The model under review builds one solid part; all positions refer to its coordinate system, in mm. A direction names the side the tool comes from. Round coordinates to 2 decimals unless told otherwise and drop trailing zeros. Order: outer loops, then holes, each group sorted by start corner. A loop starts at its lowest first (then second) coordinate and runs counter-clockwise, first axis right, second up. Notation, with made-up numbers: M -11.75,69.25 L 31.25,69.25 A25 cw 31.25,93.25 Z; hole C -18.75,-19 d9. An arc over 180 degrees is marked long. One line per item, written item: value. Start each with the question number.
from build123d import *

# Parameters (mm, degrees)
BOSS_EXTRUDE1_DEPTH     = 9
CUT_EXTRUDE1_DEPTH      = 18.867568385
CUT_EXTRUDE1_DEPTH_BACK = 18.867568385
CHAMFER1_SIZE           = 1
SKETCH4_R               = 1.25
CUT_EXTRUDE2_DEPTH      = 18.867568385
CUT_EXTRUDE3_START      = 3
SKETCH5_R               = 2.325
CUT_EXTRUDE3_DEPTH      = 10
FILLET2_R               = 2
CHAMFER3_SIZE           = 0.75


with BuildPart() as part:
    # Sketch1 → Boss-Extrude1 (new body)
    with BuildSketch(Plane.XY):
        with BuildLine():
            Line((-14, 0.5), (-14, 6.5))
            Line((-14, 6.5), (14, 6.5))
            Line((14, 6.5), (14, 0.5))
            Line((14, 0.5), (3.3, 0))
            ThreePointArc((3.3, 0), (0, 3.3), (-3.3, 0))
            Line((-3.3, 0), (-14, 0.5))
        make_face()
    extrude(amount=BOSS_EXTRUDE1_DEPTH)

    # Sketch2 → Cut-Extrude1 (cut, two sides: drawn at the far end of the back side and taken through both)
    with BuildSketch(Plane.XY.offset(9).offset(-CUT_EXTRUDE1_DEPTH_BACK)):
        Polygon((-10, 5), (0, 6.5), (-14, 6.5), (-14, 1), align=None)
        Polygon((14, 6.5), (0, 6.5), (10, 5), (14, 1), align=None)
    extrude(amount=CUT_EXTRUDE1_DEPTH + CUT_EXTRUDE1_DEPTH_BACK, mode=Mode.SUBTRACT)

    # Chamfer1
    chamfer1_edges = [part.edges().sort_by_distance(p)[0] for p in [
        (14, 0.75, 9),
        (-14, 0.75, 0),
        (-14, 0.75, 9),
        (14, 0.75, 0),
    ]]
    chamfer(chamfer1_edges, length=CHAMFER1_SIZE)

    # Sketch4 → Cut-Extrude2 (cut, through all)
    with BuildSketch(Plane(origin=(0, 0, 0), x_dir=(-1, 0, 0), z_dir=(0, 1, 0))):
        with Locations(Location((-9, 4.5, 0), (0, 0, 216.869897646))):
            Circle(SKETCH4_R)
        with Locations(Location((9, 4.5, 0), (0, 0, 323.130102354))):
            Circle(SKETCH4_R)
    extrude(amount=CUT_EXTRUDE2_DEPTH, mode=Mode.SUBTRACT)

    # Sketch5 → Cut-Extrude3 (cut)
    with BuildSketch(Plane(origin=(0, 0, 0), x_dir=(1, 0, 0), z_dir=(0, 1, 0)).offset(CUT_EXTRUDE3_START)):
        with Locations(Location((9, -4.5, 0), (0, 0, 64.525615739))):
            Circle(SKETCH5_R)
        with Locations(Location((-9, -4.5, 0), (0, 0, 115.474384261))):
            Circle(SKETCH5_R)
    extrude(amount=CUT_EXTRUDE3_DEPTH, mode=Mode.SUBTRACT)

    # Fillet2
    # the kernel refuses this fillet: 2 mm, written as the material it takes off along each edge
    with BuildSketch(Plane(origin=(10, 5, -1.647264498), x_dir=(0.7071067811865476, -0.7071067811865476, 0), z_dir=(0, 0, 1)), Plane(origin=(-10, 5, 4.048306423), x_dir=(-0.7071067811865476, -0.7071067811865476, 0), z_dir=(0, 0, -1))) as fillet2_piece_1:
        with BuildLine():
            CenterArc((FILLET2_R * 0.329452899538, -FILLET2_R), FILLET2_R, 90, 36.46923439)
            Line((-FILLET2_R * 0.264938161546, -FILLET2_R * 0.195823858534), (-FILLET2_R * 0.276825982767, -FILLET2_R * 0.179740335704))
            Line((-FILLET2_R * 0.276825982767, -FILLET2_R * 0.179740335704), (-FILLET2_R * 0.00658905799077, FILLET2_R * 0.02))
            Line((-FILLET2_R * 0.00658905799077, FILLET2_R * 0.02), (FILLET2_R * 0.329452899538, FILLET2_R * 0.02))
            Line((FILLET2_R * 0.329452899538, FILLET2_R * 0.02), (FILLET2_R * 0.329452899538, 0))
        make_face()
    extrude(amount=5.695570921, mode=Mode.SUBTRACT)
    with BuildSketch(Plane(origin=(0, 6.5, 9.75), x_dir=(0.9889363528682978, -0.1483404529302431, 0), z_dir=(0, 0, -1))) as fillet2_piece_2:
        with BuildLine():
            CenterArc((FILLET2_R * 0.15, FILLET2_R), FILLET2_R, 252.93846878, 17.06153122)
            Line((-FILLET2_R * 0.143398533007, FILLET2_R * 0.0440097799511), (-FILLET2_R * 0.149266503667, FILLET2_R * 0.0248899755501))
            Line((-FILLET2_R * 0.149266503667, FILLET2_R * 0.0248899755501), (-FILLET2_R * 0.003, -FILLET2_R * 0.02))
            Line((-FILLET2_R * 0.003, -FILLET2_R * 0.02), (FILLET2_R * 0.15, -FILLET2_R * 0.02))
            Line((FILLET2_R * 0.15, -FILLET2_R * 0.02), (FILLET2_R * 0.15, 0))
        make_face()
    extrude(amount=10.5, mode=Mode.SUBTRACT)
    with BuildSketch(Plane(origin=(-14, 1, -0.95470504), x_dir=(0, -1, 0), z_dir=(0, 0, 1))) as fillet2_piece_3:
        with BuildLine():
            CenterArc((0.861339487, 1.967087638), FILLET2_R, 225, 34.591227114)
            Line((-0.552874076, 0.552874076), (-0.581158347, 0.524589804))
            Line((-0.581158347, 0.524589804), (-0.028284271, -0.028284271))
            Line((-0.028284271, -0.028284271), (0, -0.04))
            ThreePointArc((0, -0.04), (0.25, -0.04), (0.49277321, -0.039341753))
            Line((0.49277321, -0.039341753), (0.5, 0))
        make_face()
    extrude(amount=10.90941008, mode=Mode.SUBTRACT)

    # Chamfer3
    # the kernel refuses this chamfer: 0.75 mm, written as the material it takes off along each edge
    with BuildSketch(Plane(origin=(-14.36384086, 0.63615914, 9), x_dir=(0.7068394360706732, -0.7068394360706737, 0.027495876610586747), z_dir=(0.7071067811865477, 0.7071067811865474, 0))) as chamfer3_piece_1:
        Polygon((CHAMFER3_SIZE * 0.999621916911, CHAMFER3_SIZE * 0.0274958766106), (-CHAMFER3_SIZE * 0.0274958766106, CHAMFER3_SIZE * 0.999621916911), (0, 0), align=None)
    extrude(amount=8.100165169, mode=Mode.SUBTRACT)
    with BuildSketch(Plane(origin=(-11.907423096, 4.713886536, 9), x_dir=(0.1482843679136212, -0.988562452757474, 0.027495876610586778), z_dir=(0.9889363528682975, 0.14834045293024473, 0)), Plane(origin=(0.296680906, 6.455497864, 9), x_dir=(-0.14828436791362096, -0.9885624527574741, 0.02749587661058676), z_dir=(0.9889363528682976, -0.14834045293024448, 0))) as chamfer3_piece_2:
        Polygon((CHAMFER3_SIZE * 0.999621916911, CHAMFER3_SIZE * 0.0274958766106), (-CHAMFER3_SIZE * 0.0274958766106, CHAMFER3_SIZE * 0.999621916911), (0, 0), align=None)
    extrude(amount=11.740636449, mode=Mode.SUBTRACT)
    with BuildSketch(Plane(origin=(0, 4.477625158, 9), x_dir=(0.1483404529300489, 0.9889363528683269, 0), z_dir=(0.9889363528683269, -0.1483404529300489, 0))) as chamfer3_piece_3:
        Polygon((2 - CHAMFER3_SIZE, 0), (2, -CHAMFER3_SIZE), (2, 0), align=None)
    revolve(axis=Axis((0, 4.477625158, 9), (0, 0, 1)), revolution_arc=17.06153122, mode=Mode.SUBTRACT)


solid = part.part
Item 1: Machinability: for faces 4 (the cylindrical face through (-6.734, 3.959, 3.979)), 5 (the flat face through (-11.626, 2.836, 8.63)), which of the approach directions +Z, -Z, +X, -X, +Y, -Y give a long, thin tool a straight path to every point of the face, cutting with its end or side? Answer none if there is none.
Item 2: Consider section C-C, the plane z = 5.5. Give the boundary of the cut face in (x, y), then the cut area to 3 significant figures.
Item 3: Clearance check with flat-ended pins moving along their axes: P1, Ø1, axis at x = -6.5, z = 7, coming from the -Y side; P2, Ø1.5, axis at x = -0.5, z = 2, coming from the -Y side; P3, Ø2.5, axis at x = -9.5, z = 4, coming from the +Y side. State where each tip first meets the part, or that it passes through.
Item 4: Consider section A-A, the plane z = 7.75. Give the boundary of the cut face in (x, y).
Item 5: Consider section D-D, the plane x = -1.25. Give the boundary of the cut face in (y, z).
Item 6: Consider section B-B, the plane x = -9. Give the boundary of the cut face in (y, z) (3 decimals).
Item 7: The part is to be moulded in two halves that separate along Z. For faces 1 (the cylindrical face through (9.96, 4.9, 1.33)), 2 (the flat face through (-5.16, 5.34, 8.63)), 3 (the cylindrical face through (-10.17, 1.58, 4.94)), say which applies: pulls with the +Z half, pulls with the -Z half, needs draft (parallel to the pull), parting line crosses it, or undercut.
Item 8: Wall thickness on L1, parallel to Z at x = -9, y = 0.9; L2, parallel to Z at x = 9, y = 4.2 (3 decimals); L3, parallel to X at y = 1.15, z = 4.5: over which ranges is each line inside the solid? List them lowest first.
Computed:
1. face 4: +Y
1. face 5: +Z, -X, +Y
2. outline: M -14,0.5 L -9.75,0.3 L -9.75,3 L -11.1,3 L -11.1,3.9 L -13.45,1.55 A2 ccw Z; M -8.25,0.23 L -3.3,0 A3.3 cw 3.3,0 L 8.25,0.23 L 8.25,3 L 6.9,3 L 6.9,5.46 L 0.3,6.46 A2 ccw -0.3,6.46 L -6.9,5.46 L -6.9,3 L -8.25,3 Z; M 9.75,0.3 L 14,0.5 L 14,1 L 11.1,3.9 L 11.1,3 L 9.75,3 Z
2. area: 91.2 mm^2
3. P1: stops at y = 0.13
3. P2: stops at y = 3.05
3. P3: stops at y = 3
4. outline: M -14,0.5 L -3.3,0 A3.3 cw 3.3,0 L 14,0.5 L 14,1 L 10,5 L 0.3,6.46 A2 ccw -0.3,6.46 L -10,5 L -13.45,1.55 A2 ccw Z
5. outline: M 3.05,0 L 6.31,0 L 6.31,8.25 L 5.55,9 L 3.05,9 Z
6. outline: M 0.266,0 L 5.15,0 L 5.15,2.175 L 3,2.175 L 3,3.25 L 0.266,3.25 Z; M 0.266,5.75 L 3,5.75 L 3,6.825 L 5.15,6.825 L 5.15,8.25 L 4.392,9 L 0.266,9 Z
7. face 1: needs draft
7. face 2: pulls with the +Z half
7. face 3: undercut
8. L1: z = 0 to 3.25, 5.75 to 9
8. L2: z = 0 to 2.175, 6.825 to 9
8. L3: x = -13.76 to -10.25, -7.75 to -3.09, 3.09 to 7.75, 10.25 to 13.85
